from build123d import *

# Parameters (mm, degrees)
F_4_0_4_DIAMETER_HOLE1_D     = 4
F_4_0_4_DIAMETER_HOLE1_DEPTH = 11
SKETCH4_R                    = 3
CUT_EXTRUDE1_DEPTH           = 12


with BuildPart() as part:
    # Sketch1 → Revolve1 (revolve)
    with BuildSketch(Plane.XZ):
        Polygon((25, -94), (0, -94), (0, -105), (22, -105), align=None)
    revolve(axis=Axis((0, 0, -94), (0, 0, -1)))

    # Ø4.0 (4) Diameter Hole1
    with Locations(Plane(origin=(0, 0, -105), x_dir=(-1, 0, 0), z_dir=(0, 0, -1))):
        with Locations((-14.999982566, -0.022869707), (0.022869707, -14.999982566), (-0.022869707, 14.999982566), (14.999982566, 0.022869707)):
            Hole(F_4_0_4_DIAMETER_HOLE1_D / 2, depth=F_4_0_4_DIAMETER_HOLE1_DEPTH)

    # Sketch4 → Cut-Extrude1 (cut, through all)
    with BuildSketch(Plane(origin=(0, 0, -105), x_dir=(-1, 0, 0), z_dir=(0, 0, -1))):
        Circle(SKETCH4_R)
    extrude(amount=-CUT_EXTRUDE1_DEPTH, mode=Mode.SUBTRACT)


solid = part.part
Verification items for the finished model (mm, model axes). Round coordinates to 2 decimals unless told otherwise and drop trailing zeros. Loops run counter-clockwise (first coordinate to the right, second up) from the corner with the lowest first, then second, coordinate; pieces in that order, holes last. Notation, with made-up numbers: (40.5, -30.75) - (96.5, -30.75) arc R9 ccw to (96.5, -24.75) - close; hole circle Ø11 at (-18.5, 49.5). An arc over 180 degrees is marked (long way). Answer in a Markdown table with one row per item. Add a question column.
Q1. Section check B-B on z = -98.5. Enter the section's corners in (x, y), plus the area to 3 significant figures.
Q2. Section check A-A on x = 0. Enter the section's corners in (y, z), plus the area to 3 significant figures.
Q3. Section check C-C on z = -102. Enter the section's corners in (x, y), plus the area to 3 significant figures.
Q4. Release check for a two-part mould opening along Y. For faces 1 (the face through (0, 5, -105)), 2 (the face through (21.163, -6.665, -104.312)), 3 (the face through (3, 0, -100)) record: pulls with the +Y half, pulls with the -Y half, needs draft (parallel to the pull), parting line crosses it, or undercut.
Q5. Material ranges on line 1 (Y direction, x = -15.5, z = -99.75); line 2 (X direction, y = -14, z = -97.25); line 3 (Y direction, x = 14, z = -101.25), recorded low to high.
Q6. Gauge pin test, flat ends, axial feed: pin 1 (1.5 mm diameter, centred on x = -10, z = -99.5, fed in from +Y); pin 2 (4.5 mm diameter, centred on x = -15, y = 0.02, fed in from -Z); pin 3 (5.5 mm diameter, centred on x = 0, y = 0, fed in from +Z); pin 4 (4 mm diameter, centred on y = 1, z = -102, fed in from -X). Record the tip position at first contact, or that the pin passes through.
Found:
| question | item | result |
|---|---|---|
| 1 | outline | circle Ø47.55 at (0, 0); hole circle Ø4 at (-15, 0.02); hole circle Ø6 at (0, 0); hole circle Ø4 at (-0.02, -15); hole circle Ø4 at (0.02, 15); hole circle Ø4 at (15, -0.02) |
| 1 | area | 1,700 mm² |
| 2 | outline | (-25, -94) - (-22, -105) - (-17, -105) - (-17, -94) - close; (-13, -105) - (-3, -105) - (-3, -94) - (-13, -94) - close; (3, -105) - (13, -105) - (13, -94) - (3, -94) - close; (17, -105) - (22, -105) - (25, -94) - (17, -94) - close |
| 2 | area | 363 mm² |
| 3 | outline | circle Ø45.64 at (0, 0); hole circle Ø4 at (-15, 0.02); hole circle Ø6 at (0, 0); hole circle Ø4 at (-0.02, -15); hole circle Ø4 at (0.02, 15); hole circle Ø4 at (15, -0.02) |
| 3 | area | 1,560 mm² |
| 4 | face 1 | needs draft |
| 4 | face 2 | parting line crosses it |
| 4 | face 3 | undercut |
| 5 | line 1 | y = -17.57 to -1.91, 1.96 to 17.57 |
| 5 | line 2 | x = -19.63 to -1.75, 1.71 to 19.63 |
| 5 | line 3 | y = -18.28 to -1.75, 1.71 to 18.28 |
| 6 | pin 1 | stops at y = 21.67 |
| 6 | pin 2 | stops at z = -105 |
| 6 | pin 3 | passes through |
| 6 | pin 4 | stops at x = -23.35 |
